Can you work these out from the model? Positions are in its coordinate system, mm. A direction names the side the tool comes from. Coordinates: 2 decimals unless noted, no trailing zeros. Order: outer loops, then holes, each group sorted by start corner. A loop starts at its lowest first (then second) coordinate and runs counter-clockwise, first axis right, second up. Notation, with made-up numbers: (50.25, -16) -> (76.25, -16) arc R24 ccw to (76.25, 23) -> close; hole circle Ø6 at (66, -4.75). An arc over 180 degrees is marked (long way). Return JSON: item names as keys, results as strings. Group by question number.
1) If we section it at D-D, the plane z = 2.25: Please give me the cut outline in (x, y).
2) Thinking about a two-plate mould opening in X: for faces 1 (the conical face through (-10.98, 9.84, 0.66)), 2 (the cylindrical face through (0.2, -0.1, 0.6)), 3 (the flat face through (17.5, 0, 0)), which applies, +X half, -X half, draft (parallel to the pull), parting line (faces both ways), or undercut?
3) For faces 4 (the flat face through (-17.5, 0, 0)), 5 (the cylindrical face through (-10.44, 8.15, 4.21)), which set-ups out of +Z, -Z, +X, -X, +Y, -Y let a thin tool reach every point of the face, with its end or its side?
4) If we section it at B-B, the plane y = -10.2: Please give me the cut outline in (x, z), then the cut area to 3 significant figures.
5) If we section it at A-A, the plane z = 6.25: Please give me the cut outline in (x, y), then the cut area to 3 significant figures.
6) For pin 1 (2.5 mm diameter, centred on x = -10.9, y = -10.2, fed in from -Z), with a flat end and sliding along its axis, tell me the tip position at first contact or that it passes through.
7) If I drill on probe 1 along Y at (x, z) = (10, 4.5); probe 2 along X at (y, z) = (-10.2, 1.75); probe 3 along Y at (x, z) = (10.9, 2.75), over which ranges is the centre line in solid material (lowest first)? Write a range as from..to.
from build123d import *

# Parameters (mm, degrees)
F0_W     = 35
F0_H     = 28
F1_DEPTH = 14
F3_D     = 12.8
F4_DEPTH = 7.2
F5_R     = 5
F6_D     = 3
F8_D     = 4.2
F8_DEPTH = 5.1
F8_TIP   = 1.2618073
F9_DEPTH = 2


with BuildPart() as f1:
    # F0 (on Top) → F1 (new body)
    with BuildSketch(Plane.XY):
        Rectangle(F0_W, F0_H)
    extrude(amount=F1_DEPTH)

    # F3 (through all)
    with Locations(Plane(origin=(-17.5, 0, 0), x_dir=(0, -1, 0), z_dir=(-1, 0, 0))):
        with Locations((0, 7)):
            Hole(F3_D / 2)

    # F4 (cut): a face of the model
    f4_faces = [f1.faces().sort_by_distance(p)[0] for p in [
        (0, 0, 14),
    ]]
    extrude(f4_faces, amount=-F4_DEPTH, mode=Mode.SUBTRACT)

    # F5
    f5_edges = [f1.edges().sort_by_distance(p)[0] for p in [
        (17.5, 14, 3.4),
        (-17.5, 14, 3.4),
        (17.5, -14, 3.4),
        (-17.5, -14, 3.4),
    ]]
    fillet(f5_edges, radius=F5_R)

    # F6 (through all)
    with Locations(Plane(origin=(0, 0, 0), x_dir=(1, 0, 0), z_dir=(0, 0, -1))):
        with Locations((10.9, 10.2), (-10.9, 10.2)):
            Hole(F6_D / 2)

    # F8
    with Locations(Plane.XY.offset(6.8)):
        with Locations((-10.9, 10.2), (10.9, 10.2)):
            Hole(F8_D / 2, depth=F8_DEPTH)
            with Locations((0, 0, -(F8_DEPTH + F8_TIP / 2))):  # 118° drill point
                Cone(0, F8_D / 2, F8_TIP, mode=Mode.SUBTRACT)

    # F9 (add): a face of the model
    f9_faces = [f1.faces().sort_by_distance(p)[0] for p in [
        (0, 0.15268816, 0),
    ]]
    extrude(f9_faces, amount=F9_DEPTH)


solid = f1.part
Result sheet:
{
 "1": {"outline": "(-17.5, -9) arc R5 ccw to (-12.5, -14) -> (12.5, -14) arc R5 ccw to (17.5, -9) -> (17.5, -4.29) -> (-17.5, -4.29) -> close; (-17.5, 4.29) -> (17.5, 4.29) -> (17.5, 9) arc R5 ccw to (12.5, 14) -> (-12.5, 14) arc R5 ccw to (-17.5, 9) -> close; hole circle Ø4.2 at (-10.9, 10.2); hole circle Ø3 at (-10.9, -10.2); hole circle Ø4.2 at (10.9, 10.2); hole circle Ø3 at (10.9, -10.2)"},
 "2": {"face 1": "undercut", "face 2": "draft", "face 3": "+X half"},
 "3": {"face 4": "+Z, -Z, -X, +Y, -Y", "face 5": "+Z"},
 "4": {"outline": "(-17.35, -2) -> (-12.4, -2) -> (-12.4, 6.8) -> (-17.35, 6.8) -> close; (-9.4, -2) -> (9.4, -2) -> (9.4, 6.8) -> (-9.4, 6.8) -> close; (12.4, -2) -> (17.35, -2) -> (17.35, 6.8) -> (12.4, 6.8) -> close", "area": "253 mm2"},
 "5": {"outline": "(-17.5, -9) arc R5 ccw to (-12.5, -14) -> (12.5, -14) arc R5 ccw to (17.5, -9) -> (17.5, -6.36) -> (-17.5, -6.36) -> close; (-17.5, 6.36) -> (17.5, 6.36) -> (17.5, 9) arc R5 ccw to (12.5, 14) -> (-12.5, 14) arc R5 ccw to (-17.5, 9) -> close; hole circle Ø4.2 at (-10.9, 10.2); hole circle Ø3 at (-10.9, -10.2); hole circle Ø4.2 at (10.9, 10.2); hole circle Ø3 at (10.9, -10.2)", "area": "472 mm2"},
 "6": {"pin 1": "passes through"},
 "7": {"probe 1": "y = -14..-11.4, -9..-5.89, 5.89..8.3, 12.1..14", "probe 2": "x = -17.35..-12.4, -9.4..9.4, 12.4..17.35", "probe 3": "y = -14..-11.7, -8.7..-4.79, 4.79..8.1, 12.3..14"}
}
